Work out the finished part from the listing and answer in its coordinate system (mm). Face numbers are marked on the shaded views. A direction names the side the tool comes from. Round coordinates to 2 decimals unless told otherwise and drop trailing zeros. Write each loop counter-clockwise with the first axis right and the second up, starting at its lowest first coordinate (ties: lowest second). Pieces come first, ordered by that corner, then holes. Notation, with made-up numbers: (35.25, -10.5) - (46.25, -10.5) arc R12 cw to (46.25, 3.5) - close; hole circle Ø8 at (-16, 14). An arc over 180 degrees is marked (long way). Answer as a JSON object with one key per item and string values.
Autodesk Inventor part; units mm, degrees
ref_plane "YZ Plane" through (0, 0, 0) normal (1, 0, 0) x (0, 1, 0)
ref_plane "XZ Plane" through (0, 0, 0) normal (0, 1, 0) x (-1, 0, 0)
ref_plane "XY Plane" through (0, 0, 0) normal (0, 0, 1) x (1, 0, 0)
sketch "Sketch1" plane through (0, 0, 0) normal (0, 0, 1) x (1, 0, 0)
  line L0 (0, 0) -> (-75, 0)
  line L1 (-75, 0) -> (-75, 35)
  line L2 (-75, 35) -> (0, 35)
  line L3 (0, 35) -> (0, 0)
  line L4 (3, -3) -> (-78, -3)
  line L5 (-78, -3) -> (-78, 38)
  line L6 (-78, 38) -> (3, 38)
  line L7 (3, 38) -> (3, -3)
  line L8 (-37.5, 38) -> (-37.5, 55.2273) construction
  line L9 (-78, 17.5) -> (-92.6498, 17.5) construction
  line L10 (-65, 0) -> (-65, 35)
  line L11 (-35, 0) -> (-35, 35)
  circle A0 centre (-3, 32) radius 1
  circle A1 centre (-3, 3) radius 1
  line L12 (-3, 3) -> (-3, 32) construction
  line L13 (-3, 17.5) -> (-10.1857, 17.5) construction
  circle A2 centre (-75, 35) radius 0.5
  circle A3 centre (0, 35) radius 0.5
  circle A4 centre (-75, 0) radius 0.5
  circle A5 centre (0, 0) radius 0.5
  line L14 (-75.2, 35.2) -> (-75.2, -0.2)
  line L15 (-75.2, -0.2) -> (0.2, -0.2)
  line L16 (0.2, -0.2) -> (0.2, 35.2)
  line L17 (0.2, 35.2) -> (-75.2, 35.2)
  line L18 (-65, 0) -> (-65, -1.5)
  line L19 (-65, -1.5) -> (-35, -1.5)
  line L20 (-35, -1.5) -> (-35, 0)
  point P0 (-0.5, 35)
  point P1 (0, 34.5)
  point P2 (0, 0.5)
  point P3 (-0.5, 0)
  point P4 (-75, 0.5)
  point P5 (-74.5, 0)
  point P6 (-74.5, 35)
  point P7 (-75, 34.5)
  point P8 (0.2, 0.4583)
  point P9 (0.2, 34.5417)
  point P10 (-0.4583, 35.2)
  point P11 (-74.5417, 35.2)
  point P12 (-74.5417, -0.2)
  point P13 (-0.4583, -0.2)
  point P14 (-75.2, 34.5417)
  point P15 (-75.2, 0.4583)
  point P16 (-35, -0.2)
  point P17 (-65, -0.2)
  dimension "d0" = 75
  dimension "d1" = 35
  dimension "d2" = 3
  dimension "d8" = 10
  dimension "d9" = 40
  dimension "d10" = 2
  dimension "d11" = 2
  dimension "d12" = 29
  dimension "d13" = 3
  dimension "d18" = 1
  dimension "d21" = 75
  dimension "d24" = 35
  dimension "d32" = 0.2
  dimension "d33" = 1.5
extrude "Extrusion1" add sketch "Sketch1" along normal blind 6 contours L20 L15 L18 L0 | L11 L2 A3 L3 A5 L0 | L0 L10 L2 L11 | L0 A5 L15 L20 | L18 L15 A4 L0 | L0 A4 L1 A2 L2 L10 | A5 L3 L0 | L0 L3 A5 L16 L15 | L2 A2 L17 A3 | L20 L19 L18 L15 | A4 L15 L14 L1 L0 | L0 L1 A4 | L3 A3 L16 A5 | L15 L16 A5 | A3 L17 L16 L3 L2 | L2 L3 A3 | A4 L14 A2 L1 | A4 L14 L15 | A2 L1 L2 | L2 L1 A2 L14 L17 | A3 L16 L17 | L17 L14 A2 | L4 L5 L6 L7 | A0 | A1
extrude "Extrusion2" cut sketch "Sketch1" against normal blind 1.6 from surface at 6 contours L20 L15 L18 L0 | L11 L2 A3 L3 A5 L0 | L0 L10 L2 L11 | L0 A5 L15 L20 | L18 L15 A4 L0 | L0 A4 L1 A2 L2 L10 | A5 L3 L0 | L0 L3 A5 L16 L15 | L2 A2 L17 A3 | L20 L19 L18 L15 | A4 L15 L14 L1 L0 | L0 L1 A4 | L3 A3 L16 A5 | L15 L16 A5 | A3 L17 L16 L3 L2 | L2 L3 A3 | A4 L14 A2 L1 | A4 L14 L15 | A2 L1 L2 | L2 L1 A2 L14 L17 | A3 L16 L17 | L17 L14 A2 | A0 | A1
extrude "Extrusion3" cut sketch "Sketch1" against normal blind 2 from surface at 4.4 contours L0 L10 L2 L11
extrude "Extrusion4" cut sketch "Sketch1" against normal blind 3 from surface at 4.4 contours A0 | A1
chamfer "Chamfer2" distance 1 angle 45 2 edges at (-65, -0.2, 5.2) (-35, -0.2, 5.2)
fillet "Fillet1" radius 3 4 edges at (3, 38, 3) (-78, 38, 3) (-78, -3, 3) (3, -3, 3)
ref_plane "Work Plane1" through (-37.5, 0, 0) normal (1, 0, 0) x (0, 0, -1)
sketch "Sketch2" plane through (-37.5, 0, 0) normal (1, 0, 0) x (0, 0, -1)
  line L0 (-2.4, 0) -> (-4.4, 0)
  line L1 (-4.4, 0) -> (-6, 0)
  line L2 (-6, -3) -> (-6, 0)
  line L3 (-6, -1.5) -> (-6, 0)
  line L4 (-8, -0.2) -> (-8, -1)
  line L5 (-8, -1) -> (-6, -1)
  line L6 (-8, -1) -> (-8, -1.2)
  line L7 (-8, -1.2) -> (-7.6, -1.2)
  line L8 (-7.6, -1.2) -> (-7.4, -1)
  line L9 (-8, -1) -> (-7.8322, -1.2)
  line L10 (-8, -0.2) -> (-6, -0.2)
  line L11 (-4.4, -0.2) -> (-6, -0.2)
  point P0 (0, 0)
  dimension "d41" = 0.8
  dimension "d42" = 0.2
  dimension "d45" = 45
  dimension "d46" = 50
  dimension "d47" = 0.4
  dimension "d51" = 2
ref_plane "Work Plane2" through (-67.5, 0, 0) normal (1, 0, 0) x (0, 0, -1)
extrude "Extrusion5" add sketch "Sketch2" against normal blind 1.5 from surface at -30 contours L5 L4 L10 L2 | L8 L7 L9 L5
equation "\"d11\" = d10"
equation "\"d21\" = d0"
equation "\"d24\" = d1"
properties part number "scatola_sotto"
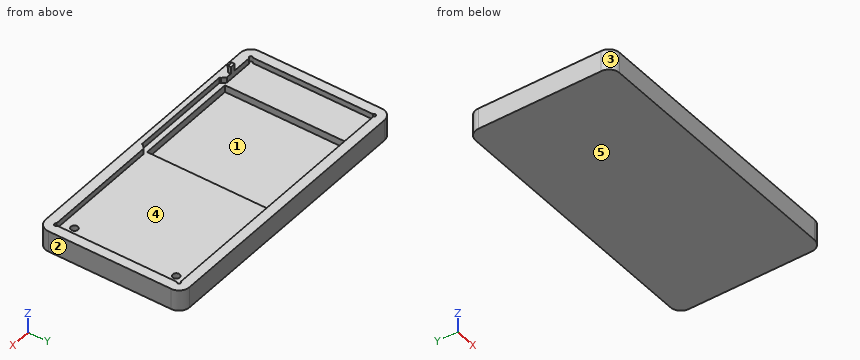
Item 1: Each of these flat-tipped pins is pushed along its axis until it touches: P1, Ø9, axis at x = -44, y = 25.5, coming from the +Z side; P2, Ø2.5, axis at x = -3, y = 3, coming from the +Z side; P3, Ø1.1, axis at y = -0.5, z = 7, coming from the -X side. Where does it stop, or does it pass through?
Results found:
{"P1": "z = 2.4", "P2": "z = 4.4", "P3": "x = -69"}
Item 2: A cutting plane is placed at A-A (y = 32). Write down the section's boundary in (x, z), and give its area (3 significant figures).
Results found:
{"outline": "(-78, 0) - (3, 0) - (3, 6) - (0.2, 6) - (0.2, 4.4) - (-2, 4.4) - (-2, 1.4) - (-4, 1.4) - (-4, 4.4) - (-35, 4.4) - (-35, 2.4) - (-65, 2.4) - (-65, 4.4) - (-75.2, 4.4) - (-75.2, 6) - (-78, 6) - close", "area": "299 mm²"}
Item 3: A cutting plane is placed at C-C (y = 10). Write down the section's boundary in (x, z).
Results found:
{"outline": "(-78, 0) - (3, 0) - (3, 6) - (0.2, 6) - (0.2, 4.4) - (-35, 4.4) - (-35, 2.4) - (-65, 2.4) - (-65, 4.4) - (-75.2, 4.4) - (-75.2, 6) - (-78, 6) - close"}
Item 4: Consider line 1 along Y through (x, z) = (-3, 3.1); line 2 along X through (y, z) = (17, 5.5); line 3 along X through (y, z) = (18, 4.25). Determine where each line is inside the solid, lowest interval first.
Results found:
{"line 1": "-3 to 2, 4 to 31, 33 to 38", "line 2": "-78 to -75.2, 0.2 to 3", "line 3": "-78 to -65, -35 to 3"}
Item 5: A cutting plane is placed at B-B (x = -3). Write down the section's boundary in (y, z), and give its area (3 significant figures).
Results found:
{"outline": "(-3, 0) - (38, 0) - (38, 6) - (35.2, 6) - (35.2, 4.4) - (33, 4.4) - (33, 1.4) - (31, 1.4) - (31, 4.4) - (4, 4.4) - (4, 1.4) - (2, 1.4) - (2, 4.4) - (-0.2, 4.4) - (-0.2, 6) - (-3, 6) - close", "area": "177 mm²"}
Item 6: For the marked faces 1 and 2, determine the directions among +Z, -Z, +X, -X, +Y, -Y from which every point of the face is accessible in a straight line to the end or side of a thin tool.
Results found:
{"face 1": "+Z", "face 2": "+Z, -Z, +X, +Y, -Y"}
Item 7: Determine the mould class of the marked faces 3, 4 and 5 for opening direction X: pulls with the +X half, pulls with the -X half, needs draft (parallel to the pull), parting line crosses it, or undercut.
Results found:
{"face 3": "pulls with the -X half", "face 4": "undercut", "face 5": "needs draft"}
